Geometry check sheet. Reference: the model listing, model coordinates, mm. Face numbers are marked on the shaded views. A direction names the side the tool comes from. Coordinates: 2 decimals unless noted, no trailing zeros. Loops run counter-clockwise (first coordinate to the right, second up) from the corner with the lowest first, then second, coordinate; pieces in that order, holes last.
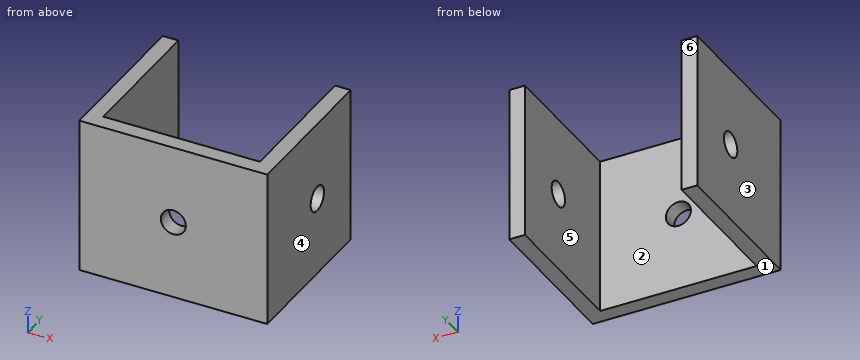
from build123d import *

# Parameters (mm, degrees)
SKETCH_1_W          = 50
SKETCH_1_H          = 50
EXTRUDE_1_DEPTH     = 5
SKETCH_2_W          = 50
SKETCH_2_H          = 50
EXTRUDE_2_DEPTH     = 5
SKETCH_3_R          = 4
CUT_EXTRUDE_1_DEPTH = 10
SKETCH_4_R          = 4
CUT_EXTRUDE_2_DEPTH = 83.006097334


with BuildPart() as part:
    # 草图1 → 凸台-拉伸1 (new body)
    with BuildSketch(Plane(origin=(0, 0, 0), x_dir=(1, 0, 0), z_dir=(0, 1, 0))):
        Rectangle(SKETCH_1_W, SKETCH_1_H)
    extrude(amount=EXTRUDE_1_DEPTH)

    # 草图2 → 凸台-拉伸2 (add)
    with BuildSketch(Plane(origin=(25, 0, 0), x_dir=(0, 0, -1), z_dir=(1, 0, 0))):
        with Locations((0, 25)):
            Rectangle(SKETCH_2_W, SKETCH_2_H)
    extrude_2 = extrude(amount=EXTRUDE_2_DEPTH)

    # 镜向1: 凸台-拉伸2 across plane
    add(extrude_2.mirror(Plane(origin=(0, 0, 0), x_dir=(0, 0, 1), z_dir=(1, 0, 0))))

    # 草图3 → 切除-拉伸1 (cut)
    with BuildSketch(Plane(origin=(0, 5, 0), x_dir=(1, 0, 0), z_dir=(0, 1, 0))):
        with Locations(Location((0, 0, 0), (0, 0, 270))):
            Circle(SKETCH_3_R)
    extrude(amount=-CUT_EXTRUDE_1_DEPTH, mode=Mode.SUBTRACT)

    # 草图4 → 切除-拉伸2 (cut, through all)
    with BuildSketch(Plane(origin=(30, 0, 0), x_dir=(0, 0, -1), z_dir=(1, 0, 0))):
        with Locations((0, 30)):
            Circle(SKETCH_4_R)
    extrude(amount=-CUT_EXTRUDE_2_DEPTH, mode=Mode.SUBTRACT)


solid = part.part
1) Section check C-C on x = 0. Record the cut outline in (y, z).
Data:
outline: (0, -25) - (5, -25) - (5, -4) - (0, -4) - close; (0, 4) - (5, 4) - (5, 25) - (0, 25) - close
2) Depth check by flat-ended pin: pin 1 (3 mm diameter, centred on x = 9, z = 2, fed in from +Y). Enter the tip coordinate at first touch or a pass-through.
Data:
pin 1: stops at y = 5
3) Access from +Z, -Z, +X, -X, +Y, -Y to the whole of each face (thin tool, end or side, straight path). Record for the marked faces 1 and 2.
Data:
face 1: -Z, +X, -X, +Y, -Y
face 2: +Z, -Z, +Y
4) Section check A-A on z = 0. Record the cut outline in (x, y), and give its area (3 significant figures).
Data:
outline: (-30, 0) - (-4, 0) - (-4, 5) - (-25, 5) - (-25, 26) - (-30, 26) - close; (-30, 34) - (-25, 34) - (-25, 50) - (-30, 50) - close; (4, 0) - (30, 0) - (30, 26) - (25, 26) - (25, 5) - (4, 5) - close; (25, 34) - (30, 34) - (30, 50) - (25, 50) - close
area: 630 mm2
5) Section check D-D on y = 42. Record the cut outline in (x, z), and give its area (3 significant figures).
Data:
outline: (-30, -25) - (-25, -25) - (-25, 25) - (-30, 25) - close; (25, -25) - (30, -25) - (30, 25) - (25, 25) - close
area: 500 mm2
6) Material ranges on probe 1 along X at (y, z) = (8, 22); probe 2 along X at (y, z) = (3.6, 0); probe 3 along Y at (x, z) = (26, 0), recorded low to high.
Data:
probe 1: x = -30 to -25, 25 to 30
probe 2: x = -30 to -4, 4 to 30
probe 3: y = 0 to 26, 34 to 50
7) Mould release check, pull along X, two halves, no side actions. Record for the marked faces 3, 4, 5 and 6: +X half, -X half, draft (parallel to the pull), parting line (faces both ways), or undercut.
Data:
face 3: -X half
face 4: +X half
face 5: undercut
face 6: draft
8) Section check B-B on y = 30. Record the cut outline in (x, z).
Data:
outline: (-30, -25) - (-25, -25) - (-25, -4) - (-30, -4) - close; (-30, 4) - (-25, 4) - (-25, 25) - (-30, 25) - close; (25, -25) - (30, -25) - (30, -4) - (25, -4) - close; (25, 4) - (30, 4) - (30, 25) - (25, 25) - close
